Source: three-view drawing plus pictorial views. Frame: mm from the lowest corner of the part. Give positions to 0.01 mm unless a question says otherwise; leave off trailing zeros. Loops run counter-clockwise (first coordinate to the right, second up) from the corner with the lowest first, then second, coordinate; pieces in that order, holes last. Notation, with made-up numbers: (16, 9.25) -> (43, 9.25) arc R20 ccw to (43, 42.25) -> close; hole circle Ø10 at (8, 9). An arc over 180 degrees is marked (long way). Put each result on its own line as item: value.
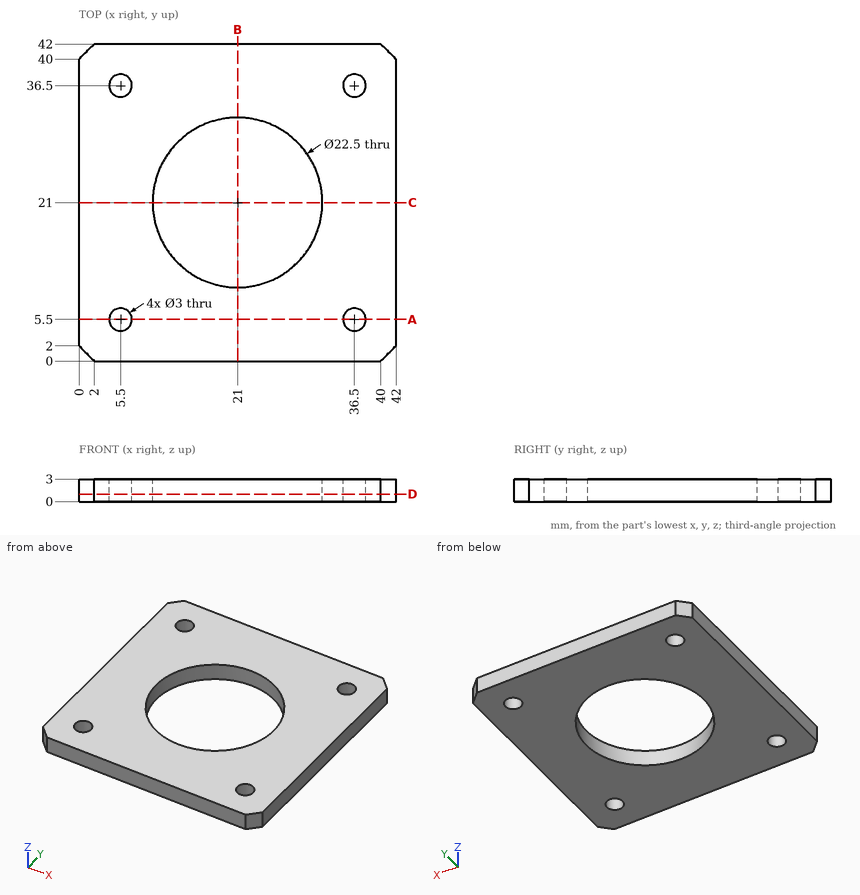
(1) Line query: probe 1 along X at (y, z) = (36.5, 1.65); probe 2 along Y at (x, z) = (21, 2.05). Output: solid intervals per line, ascending. Write a range as from..to.
Calculated:
probe 1: x = 0..4, 7..35, 38..42
probe 2: y = 0..9.75, 32.25..42
(2) Section A-A on y = 5.5. Return loops of the section in (x, z).
Calculated:
outline: (0, 0) -> (4, 0) -> (4, 3) -> (0, 3) -> close; (7, 0) -> (35, 0) -> (35, 3) -> (7, 3) -> close; (38, 0) -> (42, 0) -> (42, 3) -> (38, 3) -> close
(3) Section B-B on x = 21. Return loops of the section in (y, z).
Calculated:
outline: (0, 0) -> (9.75, 0) -> (9.75, 3) -> (0, 3) -> close; (32.25, 0) -> (42, 0) -> (42, 3) -> (32.25, 3) -> close
(4) Section D-D on z = 1. Return loops of the section in (x, y).
Calculated:
outline: (0, 2) -> (2, 0) -> (40, 0) -> (42, 2) -> (42, 40) -> (40, 42) -> (2, 42) -> (0, 40) -> close; hole circle Ø3 at (5.5, 5.5); hole circle Ø3 at (5.5, 36.5); hole circle Ø22.5 at (21, 21); hole circle Ø3 at (36.5, 5.5); hole circle Ø3 at (36.5, 36.5)
